Job drawing, mm, ordinate dimensions from the low corner. One solid piece. A direction names the side the tool comes from. Give positions to 0.01 mm unless a question says otherwise; leave off trailing zeros. Write each loop counter-clockwise with the first axis right and the second up, starting at its lowest first coordinate (ties: lowest second). Pieces come first, ordered by that corner, then holes. Notation, with made-up numbers: M -10,77.5 L 22,77.5 A14 ccw 22,88.5 Z; hole C 38,41.25 d2. An arc over 180 degrees is marked long. Answer as CSV lines item,"result". Start each with the question number.
Item 1: Band-saw the part on C-C, the plane z = 31. List the corners of the cut face in (x, y).
Item 2: Band-saw the part on D-D, the plane z = 14. List the corners of the cut face in (x, y).
Item 3: Pin check, flat tips, straight feed: pin 1 (6 mm diameter, centred on x = 25, z = 45, fed in from -Y); pin 2 (9 mm diameter, centred on y = 16.5, z = 32.5, fed in from +X); pin 3 (12 mm diameter, centred on y = 16.5, z = 50, fed in from -X); pin 4 (1 mm diameter, centred on x = 62, y = 17.5, fed in from +Z). Stop position of each tip, or through.
Item 4: Band-saw the part on B-B, the plane x = 61. List the corners of the cut face in (y, z), then the cut area to 3 significant figures.
Item 5: Band-saw the part on A-A, the plane y = 47. List the corners of the cut face in (x, z).
Item 6: 3-axis set-ups, long thin cutter, end or side, ignore diameter. For the marked faces 1, 2 and 3: which of +Z, -Z, +X, -X, +Y, -Y reach the whole face in a straight line?
Item 7: Wall check: L1, parallel to X at y = 51, z = 9.5; L2, parallel to X at y = 7, z = 41; L3, parallel to Z at x = 52, y = 3.5. Give the ranges that are in metal, low to high. Write a range as from..to.
Item 8: Two-plate mould, pull along X, no slides. Class the marked faces 4, 5, 6 and 7: +X half, -X half, draft (parallel to the pull), parting line (faces both ways), or undercut.
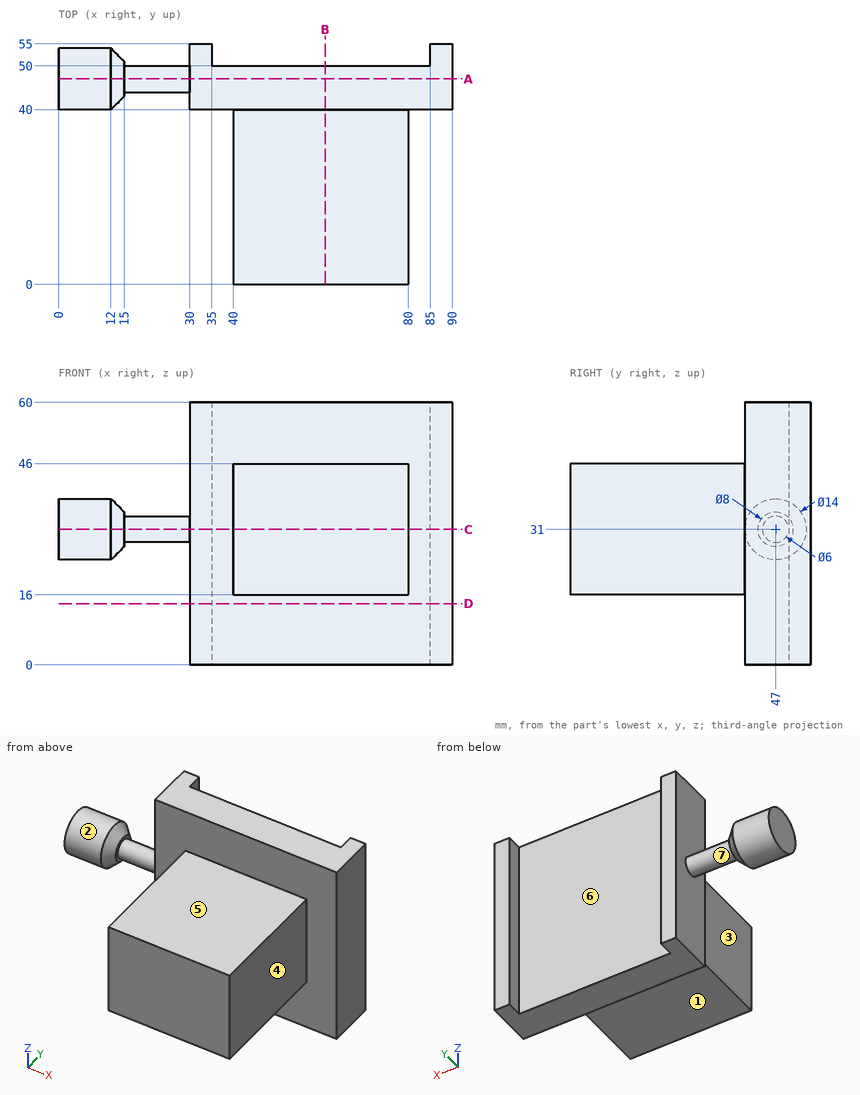
Output:
1,outline,"M 0,40 L 12,40 L 15,43 L 15,44 L 30,44 L 30,40 L 40,40 L 40,0 L 80,0 L 80,40 L 90,40 L 90,55 L 85,55 L 85,50 L 35,50 L 35,55 L 30,55 L 30,50 L 15,50 L 15,51 L 12,54 L 0,54 Z"
2,outline,"M 30,40 L 90,40 L 90,55 L 85,55 L 85,50 L 35,50 L 35,55 L 30,55 Z"
3,pin 1,"through"
3,pin 2,"x = 80"
3,pin 3,"x = 40"
3,pin 4,"z = 46"
4,outline,"M 0,16 L 40,16 L 40,0 L 50,0 L 50,60 L 40,60 L 40,46 L 0,46 Z"
4,area,"1,800 mm²"
5,outline,"M 0,24 L 12,24 L 15,27 L 15,28 L 30,28 L 30,0 L 90,0 L 90,60 L 30,60 L 30,34 L 15,34 L 15,35 L 12,38 L 0,38 Z"
6,face 1,"-Z, +X, -X, -Y"
6,face 2,"-X"
6,face 3,"+Z, -Z, -X, -Y"
7,L1,"30..35, 85..90"
7,L2,"40..80"
7,L3,"16..46"
8,face 4,"+X half"
8,face 5,"draft"
8,face 6,"undercut"
8,face 7,"undercut"
